Autodesk Inventor part; units mm, degrees
ref_plane "YZ Plane" through (0, 0, 0) normal (1, 0, 0) x (0, 1, 0)
ref_plane "XZ Plane" through (0, 0, 0) normal (0, 1, 0) x (-1, 0, 0)
ref_plane "XY Plane" through (0, 0, 0) normal (0, 0, 1) x (1, 0, 0)
sketch "Sketch1" plane through (0, 0, 0) normal (0, 0, 1) x (1, 0, 0)
  line L0 (0, 0) -> (82.3, 0)
  line L1 (82.3, 0) -> (82.3, 20)
  line L2 (82.3, 20) -> (0, 20)
  line L3 (0, 20) -> (0, 0)
  line L4 (-2.8173, 10) -> (83.4818, 10)
  line L5 (41.15, 24.9256) -> (41.15, -5.5134)
  line L6 (41.15, -5.5134) -> (20, -5.5134) construction
  line L7 (41.15, -5.5134) -> (62.3, -5.5134) construction
  line L8 (20, -5.5134) -> (20, 27.3565) construction
  line L9 (62.3, -5.5134) -> (62.3, 27.7135) construction
  line L10 (20, -5.5134) -> (10, -5.5134) construction
  line L11 (10, -5.5134) -> (10, 28.7251)
  circle A0 centre (10, 10) radius 3
  line L12 (20, -5.5134) -> (30, -5.5134) construction
  line L13 (30, -5.5134) -> (30, 27.7135)
  circle A1 centre (30, 10) radius 3
  line L14 (62.3, -5.5134) -> (72.3, -5.5134) construction
  line L15 (72.3, -5.5134) -> (72.3, 24.2533)
  line L16 (62.3, -5.5134) -> (52.3, -5.5134)
  line L17 (52.3, -5.5134) -> (52.3, 29.0456)
  circle A2 centre (52.3, 10) radius 3
  circle A3 centre (72.3, 10) radius 3
  dimension "d0" = 82.3
  dimension "d1" = 20
  dimension "d2" = 21.15
  dimension "d3" = 21.15
  dimension "d4" = 10
  dimension "d5" = 6
  dimension "d6" = 10
  dimension "d7" = 6
  dimension "d8" = 10
  dimension "d9" = 10
  dimension "d10" = 6
  dimension "d11" = 6
extrude "Extrusion1" add sketch "Sketch1" along normal blind 5 contours L3 L4 A0 L11 L0 | L11 A0 L4 A1 L13 L0 | L3 L2 L11 A0 L4 | L13 A1 L4 L5 L0 | L5 L4 A2 L17 L0 | A0 L11 L2 L13 A1 L4 | L17 A2 L4 A3 L15 L0 | L5 L2 L17 A2 L4 | L4 A1 L13 L2 L5 | L15 A3 L4 L1 L0 | A2 L17 L2 L15 A3 L4 | L4 A3 L15 L2 L1
sketch "Sketch2" plane through (0, 20, 0) normal (0, 1, 0) x (1, 0, 0)
  line L0 (82.3, 0) -> (0, 0)
  line L1 (0, 0) -> (0, -5)
  line L2 (82.3, 0) -> (82.3, -5)
  line L3 (41.15, 64.2436) -> (41.15, -26.8176)
  line L4 (41.15, 0) -> (66.15, 0)
  line L5 (66.15, 0) -> (66.15, 50)
  line L6 (66.15, 50) -> (16.15, 50)
  line L7 (16.15, 50) -> (16.15, 0)
  circle A0 centre (41.15, 25) radius 11
  line L8 (41.15, 64.2436) -> (57.65, 64.2436)
  line L9 (57.65, 6.1421) -> (5.0097, 6.1421)
  circle A1 centre (57.65, 41.5) radius 1.6
  circle A2 centre (24.65, 41.5) radius 1.6
  circle A3 centre (24.65, 10.5) radius 1.6
  circle A4 centre (57.65, 10.5) radius 1.6
  dimension "d14" = 25
  dimension "d15" = 50
  dimension "d16" = 50
  dimension "d17" = 22
  dimension "d20" = 16.5
  dimension "d22" = 3.2
  dimension "d23" = 3.2
  dimension "d24" = 3.2
  dimension "d25" = 3.2
extrude "Extrusion2" add sketch "Sketch2" against normal blind 5 contours L0 L3 A0 L6 L5 | L0 L7 L9 L3 | L9 L7 L6 L3 A0
sketch "Sketch3" plane through (16.15, 20, -50) normal (-1, 0, 0) x (0, 0, 1)
  line L0 (50, -5) -> (0, -5)
  line L1 (50, 0) -> (50, -5)
  line L2 (1.2041, -5) -> (50, -20)
  line L3 (50, -20) -> (50, -5)
  line L4 (50, -20) -> (50, -5)
  line L5 (50, -5) -> (1.2041, -5)
extrude "Extrusion3" add sketch "Sketch3" against normal blind 3
sketch "Sketch4" plane through (66.15, 20, 0) normal (1, 0, 0) x (0, 0, -1)
  line L0 (50, -5) -> (0, -5)
  line L1 (0, -20) -> (50, -5)
  line L2 (50, -5) -> (1.261, -5)
  line L3 (0, -5) -> (0, -20)
extrude "Extrusion4" add sketch "Sketch4" against normal blind 3
properties part number "z motor mount" material "ABS Plastic"
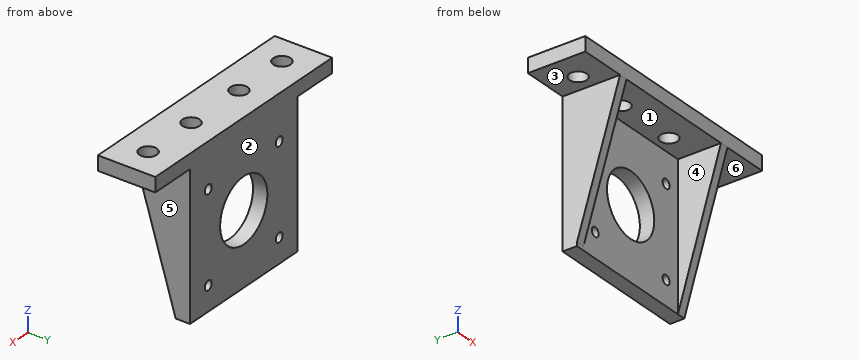
For this review, take the finished solid that the model builds, in its own axes (mm). Face numbers are marked on the shaded views. A direction names the side the tool comes from. Round coordinates to 2 decimals unless told otherwise and drop trailing zeros. Write each loop counter-clockwise with the first axis right and the second up, starting at its lowest first coordinate (ties: lowest second). Pieces come first, ordered by that corner, then holes. Notation, with made-up numbers: (20.5, 46.5) - (37.5, 46.5) arc R34 ccw to (37.5, 79.5) - close; hole circle Ø5 at (18, 74.25). An arc over 180 degrees is marked (long way). Write item = value, one per line. Start each with the question number.
1. Draft analysis for pull direction X (two halves, no side actions). For the marked faces 4, 5 and 6, state which applies: released by +X, released by -X, zero draft, split by the parting line, or undercut.
2. Consider section B-B on x = 10. State the section outline as (y, z) points, plus the area to 3 significant figures.
3. Wall thickness on L1, parallel to X at y = 10, z = 3.3; L2, parallel to X at y = 17.95, z = -41.5; L3, parallel to Z at x = 57.65, y = 17.3: over which ranges is each line inside the solid? List them lowest first.
4. Consider section A-A on x = 57.65. State the section outline as (y, z) points.
5. Consider section D-D on z = -41.5. State the section outline as (x, y) points.
6. For the marked faces 1, 2 and 3, list the 3-axis set-ups (+Z, -Z, +X, -X, +Y, -Y) from which the entire face can be reached by the end or side of a thin tool; tool diameter is ignored.
7. Consider section C-C on y = 16.5. State the section outline as (x, z) points.
8. For pin 1 Ø5 at (x, y) = (11, 11) entering from -Z; pin 2 Ø10 at (y, z) = (13.5, -17.5) entering from +X; pin 3 Ø12 at (y, z) = (8.5, -37) entering from -X, all flat-tipped, find the tip position at first contact; note any pin that passes through.
Evaluation:
q1.face_4 = undercut
q1.face_5 = released by +X
q1.face_6 = zero draft
q2.outline = (0, 0) - (7, 0) - (7, 5) - (0, 5) - close; (13, 0) - (20, 0) - (20, 5) - (13, 5) - close
q2.area = 70.0 mm2
q3.L1 = 0 to 7, 13 to 27, 33 to 49.3, 55.3 to 69.3, 75.3 to 82.3
q3.L2 = 16.15 to 23.05, 26.25 to 56.05, 59.25 to 66.15
q3.L3 = -50 to -43.1, -39.9 to -12.1, -8.9 to 5
q4.outline = (0, 0) - (15, 0) - (15, -8.9) - (20, -8.9) - (20, 5) - (0, 5) - close; (15, -50) - (20, -50) - (20, -43.1) - (15, -43.1) - close; (15, -39.9) - (20, -39.9) - (20, -12.1) - (15, -12.1) - close
q5.outline = (16.15, 12.76) - (19.15, 12.76) - (19.15, 15) - (23.05, 15) - (23.05, 20) - (16.15, 20) - close; (26.25, 15) - (56.05, 15) - (56.05, 20) - (26.25, 20) - close; (59.25, 15) - (63.15, 15) - (63.15, 12.45) - (66.15, 12.45) - (66.15, 20) - (59.25, 20) - close
q6.face_1 = -Z, -Y
q6.face_2 = +Z, -Z, +X, -X, +Y
q6.face_3 = -Z, -X, +Y, -Y
q7.outline = (0, 0) - (16.15, 0) - (16.15, -50) - (66.15, -50) - (66.15, 0) - (82.3, 0) - (82.3, 5) - (0, 5) - close; hole circle Ø3.2 at (24.65, -41.5); hole circle Ø3.2 at (24.65, -10.5); hole circle Ø22 at (41.15, -25); hole circle Ø3.2 at (57.65, -41.5); hole circle Ø3.2 at (57.65, -10.5)
q8.pin_1 = 0
q8.pin_2 = 66.15
q8.pin_3 = 16.15
